Geometry: final body of the model. Coordinates: model frame, mm. Face numbers are marked on the shaded views. A direction names the side the tool comes from. Give positions to 0.01 mm unless a question says otherwise; leave off trailing zeros. Write each loop counter-clockwise with the first axis right and the second up, starting at its lowest first coordinate (ties: lowest second). Pieces come first, ordered by that corner, then holes. Notation, with made-up numbers: (8.5, -22.75) -> (57.5, -22.75) arc R15 ccw to (57.5, -3.75) -> close; hole circle Ø9 at (82.5, 30). An arc over 180 degrees is marked (long way). Answer in a Markdown table with one row per item. Add a question column.
from build123d import *

# Parameters (mm, degrees)
F0_W     = 20
F0_H     = 20
F0_W_2   = 550
F0_H_2   = 360
F1_DEPTH = 280
F2_DEPTH = 300


with BuildPart() as f1:
    # F0 (on Top) → F1 (new body)
    with BuildSketch(Plane.XY):
        with Locations((-285, 190)):
            Rectangle(F0_W, F0_H)
        with Locations((285, 190)):
            Rectangle(F0_W, F0_H)
        with Locations((0, 190)):
            Rectangle(F0_W_2, F0_H)
        with Locations((-285, 0)):
            Rectangle(F0_W, F0_H_2)
        with Locations((285, 0)):
            Rectangle(F0_W, F0_H_2)
    extrude(amount=F1_DEPTH)

    # F0 (on Top) → F2 (join)
    with BuildSketch(Plane.XY):
        with Locations((-285, -190)):
            Rectangle(F0_W, F0_H)
        with Locations((0, -190)):
            Rectangle(F0_W_2, F0_H)
        with Locations((285, -190)):
            Rectangle(F0_W, F0_H)
    extrude(amount=F2_DEPTH)


solid = f1.part
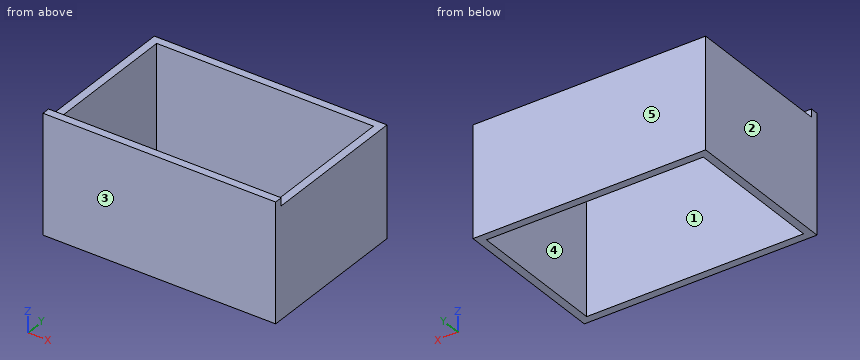
Q1. Line query: probe 1 along X at (y, z) = (163.5, 33); probe 2 along Y at (x, z) = (142, 275). Output: solid intervals per line, ascending. Write a range as from..to.
Q2. Access query for the marked faces 4 and 5. Directions: +Z, -Z, +X, -X, +Y, -Y. A direction counts if a zero-diameter tool reaches every point of the face in a straight line with its end or side. Return the directions, or none.
Q3. Section A-A on x = 117.5. Return loops of the section in (y, z), and give its area (3 significant figures).
Q4. Section B-B on y = 159. Return loops of the section in (x, z).
Q5. Section C-C on z = 212. Return loops of the section in (x, y), and give its area (3 significant figures).
Q6. Pull-direction query (Y, two-part tool) for the marked faces 1, 2 and 3; classes: +Y half, -Y half, draft (parallel to the pull), parting line (faces both ways), or undercut.
Checks:
| question | item | result |
|---|---|---|
| 1 | probe 1 | -295..-275, 275..295 |
| 1 | probe 2 | -200..-180, 180..200 |
| 2 | face 4 | +Z, -Z |
| 2 | face 5 | +Z, -Z, +X, -X, +Y |
| 3 | outline | (-200, 0) -> (-180, 0) -> (-180, 300) -> (-200, 300) -> close; (180, 0) -> (200, 0) -> (200, 280) -> (180, 280) -> close |
| 3 | area | 11,600 mm^2 |
| 4 | outline | (-295, 0) -> (-275, 0) -> (-275, 280) -> (-295, 280) -> close; (275, 0) -> (295, 0) -> (295, 280) -> (275, 280) -> close |
| 5 | outline | (-295, -200) -> (295, -200) -> (295, 200) -> (-295, 200) -> close; hole (-275, -180) -> (275, -180) -> (275, 180) -> (-275, 180) -> close |
| 5 | area | 38,000 mm^2 |
| 6 | face 1 | undercut |
| 6 | face 2 | draft |
| 6 | face 3 | -Y half |
